from build123d import *

# Parameters (mm, degrees)
BOSS_EXTRUDE1_DEPTH = 12
SKETCH3_R           = 1.5
CUT_EXTRUDE1_DEPTH  = 70.883402894
SKETCH4_R           = 1.5
CUT_EXTRUDE3_DEPTH  = 72.291233683
SKETCH6_OUTSIDE_W   = 47.446
SKETCH6_OUTSIDE_H   = 41.446
CUT_EXTRUDE4_DEPTH  = 95.687327558
FILLET1_R           = 5
FILLET2_R           = 5
FILLET3_R           = 5
FILLET4_R           = 1.1
FILLET5_R           = 1.1
CUT_EXTRUDE5_DEPTH  = 70.883402894
FILLET6_R           = 2
FILLET7_R           = 2
FILLET8_R           = 2
FILLET9_R           = 2


with BuildPart() as part:
    # Sketch2 → Boss-Extrude1 (new, symmetric)
    with BuildSketch(Plane.XY):
        Polygon((-13.986484746, 65.5), (0, 0), (8.8, 0), (8.8, -1.5), (-1.213515254, -1.5), (-15.2, 64), (-21.2, 64), (-21.2, 65.5), align=None)
    extrude(amount=BOSS_EXTRUDE1_DEPTH, both=True)

    # Sketch3 → Cut-Extrude1 (cut, through all)
    with BuildSketch(Plane(origin=(0, 0, 0), x_dir=(1, 0, 0), z_dir=(0, 1, 0))):
        with Locations(Location((3.8, 9, 0), (0, 0, 270))):
            Circle(SKETCH3_R)
        with Locations(Location((3.8, -9, 0), (0, 0, 270))):
            Circle(SKETCH3_R)
    extrude(amount=-CUT_EXTRUDE1_DEPTH, mode=Mode.SUBTRACT)

    # Sketch4 → Cut-Extrude3 (cut, through all)
    with BuildSketch(Plane(origin=(0, 65.5, 0), x_dir=(1, 0, 0), z_dir=(0, 1, 0))):
        with Locations(Location((-18.2, 0, 0), (0, 0, 270))):
            Circle(SKETCH4_R)
    extrude(amount=-CUT_EXTRUDE3_DEPTH, mode=Mode.SUBTRACT)

    # Sketch6 outside → Cut-Extrude4 (cut, through all)
    with BuildSketch(Plane(origin=(0, 90, 0), x_dir=(1, 0, 0), z_dir=(0, 1, 0))):
        with Locations((-6.2, 0)):
            Rectangle(SKETCH6_OUTSIDE_W, SKETCH6_OUTSIDE_H)
        Polygon((-21.2, 6), (-13.986484746, 6), (0, 12), (8.8, 12), (8.8, -12), (0, -12), (-13.986484746, -6), (-21.2, -6), align=None, mode=Mode.SUBTRACT)
    extrude(amount=-CUT_EXTRUDE4_DEPTH, mode=Mode.SUBTRACT)

    # Fillet1
    fillet1_edges = [part.edges().sort_by_distance(p)[0] for p in [
        (8.8, -0.75, 12),
    ]]
    fillet(fillet1_edges, radius=FILLET1_R)

    # Fillet2
    fillet2_edges = [part.edges().sort_by_distance(p)[0] for p in [
        (8.8, -0.75, -12),
    ]]
    fillet(fillet2_edges, radius=FILLET2_R)

    # Fillet3
    fillet3_edges = [part.edges().sort_by_distance(p)[0] for p in [
        (-21.2, 64.75, 6),
        (-21.2, 64.75, -6),
    ]]
    fillet(fillet3_edges, radius=FILLET3_R)

    # Fillet4
    fillet4_edges = [part.edges().sort_by_distance(p)[0] for p in [
        (-1.213515254, -1.5, 0),
    ]]
    fillet(fillet4_edges, radius=FILLET4_R)

    # Fillet5
    fillet5_edges = [part.edges().sort_by_distance(p)[0] for p in [
        (-13.986484746, 65.5, 0),
    ]]
    fillet(fillet5_edges, radius=FILLET5_R)

    # Sketch7 → Cut-Extrude5 (cut, through all)
    with BuildSketch(Plane(origin=(0, 0, 0), x_dir=(0, 0, -1), z_dir=(0.9779527521078789, 0.20882627862562123, 0))):
        Polygon((-6.757100422, 13.69539962), (6.201245399, 13.69539962), (1.722072489, 63.69539962), (-2.277927511, 63.69539962), align=None)
    extrude(amount=-CUT_EXTRUDE5_DEPTH, mode=Mode.SUBTRACT)

    # Fillet6
    fillet6_edges = [part.edges().sort_by_distance(p)[0] for p in [
        (-14.034737832, 62.134471646, -1.722072489),
    ]]
    fillet(fillet6_edges, radius=FILLET6_R)

    # Fillet7
    fillet7_edges = [part.edges().sort_by_distance(p)[0] for p in [
        (-14.034737832, 62.134471646, 2.277927511),
    ]]
    fillet(fillet7_edges, radius=FILLET7_R)

    # Fillet8
    fillet8_edges = [part.edges().sort_by_distance(p)[0] for p in [
        (-3.593423901, 13.236834041, -6.201245399),
    ]]
    fillet(fillet8_edges, radius=FILLET8_R)

    # Fillet9
    fillet9_edges = [part.edges().sort_by_distance(p)[0] for p in [
        (-3.593423901, 13.236834041, 6.757100422),
    ]]
    fillet(fillet9_edges, radius=FILLET9_R)


solid = part.part
Here's how the part is built. I have some questions about the finished solid (model axes, mm). A direction names the side the tool comes from. Round coordinates to 2 decimals unless told otherwise and drop trailing zeros. Write each loop counter-clockwise with the first axis right and the second up, starting at its lowest first coordinate (ties: lowest second). Pieces come first, ordered by that corner, then holes. Notation, with made-up numbers: (25, 71) -> (36, 71) arc R4 ccw to (36, 75) -> close; hole circle Ø10 at (65, 51). An arc over 180 degrees is marked (long way). One line per item, written item: value.
1) We'd pull the mould along Z, two halves only. Please class faces 1 (the face through (-3.743, 13.888, -5.506)), 2 (the face through (-15, 64, 6)), 3 (the face through (-16.8, 64, -1.2)): released by +Z, released by -Z, zero draft, split by the parting line, or undercut.
Filled sheet:
face 1: undercut
face 2: released by +Z
face 3: zero draft
2) Suppose I cut it at A-A on z = 8.25. List the corners of the cut face in (x, y) for me.
Filled sheet:
outline: (-8.74, 33.75) -> (-1.4, -0.63) arc R1.1 ccw to (-0.32, -1.5) -> (2.5, -1.5) -> (2.5, 0) -> (0, 0) -> (-8.74, 40.94) -> close; (5.1, -1.5) -> (8.64, -1.5) -> (8.64, 0) -> (5.1, 0) -> close
3) If I drill on line 1 (Y direction, x = 2, z = 6); line 2 (Y direction, x = -17, z = -3.75); line 3 (X direction, y = 64.75, z = 0), over which ranges is the centre line in solid material (lowest first)? Write a range as [from, to].
Filled sheet:
line 1: y = [-1.5, 0]
line 2: y = [64, 65.5]
line 3: x = [-21.2, -19.7], [-16.7, -13.83]
4) Suppose I cut it at C-C on x = -18.2. List the corners of the cut face in (y, z) for me, plus the area to 3 significant figures.
Filled sheet:
outline: (64, -5.58) -> (65.5, -5.58) -> (65.5, -1.5) -> (64, -1.5) -> close; (64, 1.5) -> (65.5, 1.5) -> (65.5, 5.58) -> (64, 5.58) -> close
area: 12.2 mm2
5) For faces 4 (the face through (7.37, -0.76, -10.5)), 5 (the face through (-15, 64, -6)), 6 (the face through (-13.938, 61.633, 1.783)), which set-ups out of +Z, -Z, +X, -X, +Y, -Y let a thin tool reach every point of the face, with its end or its side?
Filled sheet:
face 4: -Z, +X, +Y, -Y
face 5: -Z, -X, +Y, -Y
face 6: +X, -Y
6) Suppose I cut it at B-B on y = 37.5. List the corners of the cut face in (x, z) for me, plus the area to 3 significant figures.
Filled sheet:
outline: (-9.54, -7.91) -> (-8.01, -8.56) -> (-8.01, -3.99) -> (-9.54, -3.96) -> close; (-9.54, 4.52) -> (-8.01, 4.55) -> (-8.01, 8.56) -> (-9.54, 7.91) -> close
area: 12.2 mm2
7) I'm going to push flat-ended pins straight in: pin 1 Ø1.8 at (x, y) = (-15, 63) entering from -Z; pin 2 Ø3 at (y, z) = (9, -8) entering from -X; pin 3 Ø3 at (x, z) = (-17.5, -1.5) entering from -Y. Where does each tip first touch, or does it pass through?
Filled sheet:
pin 1: stops at z = -6
pin 2: stops at x = -3.78
pin 3: stops at y = 64
